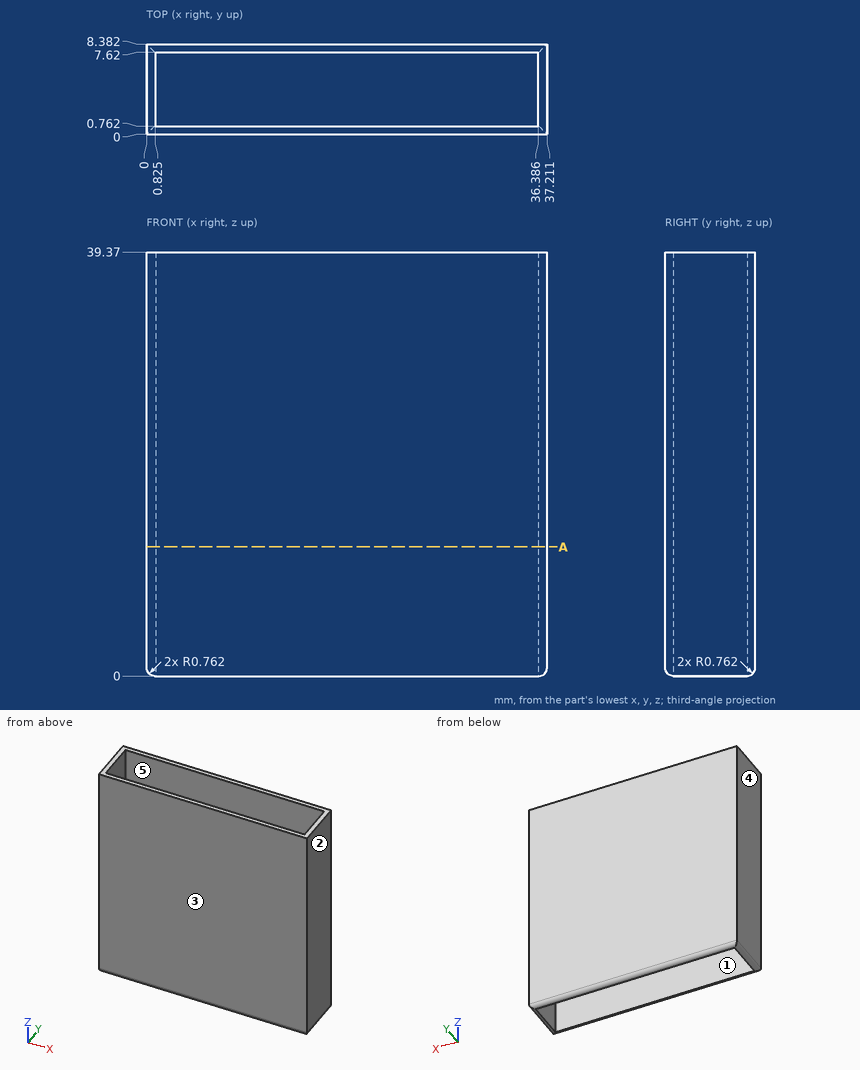
The figure shows three views and two pictorial views of one solid part (mm, origin at its lowest corner). Answer the questions. A direction names the side the tool comes from. Round coordinates to 2 decimals unless told otherwise and drop trailing zeros. Loops run counter-clockwise (first coordinate to the right, second up) from the corner with the lowest first, then second, coordinate; pieces in that order, holes last. Notation, with made-up numbers: (58, 34) - (117, 34) arc R23 cw to (117, 60) - close; hole circle Ø5 at (76.25, 48.25). An arc over 180 degrees is marked (long way). Use one line per item in the form item = value. Start each with the question number.
(1) Determine the mould class of the marked faces 1, 2 and 3 for opening direction X: +X half, -X half, draft (parallel to the pull), parting line (faces both ways), or undercut.
(2) Which of the six approach directions +Z, -Z, +X, -X, +Y, -Y give full straight-line access (tool end or side, diameter ignored) to the marked faces 4 and 5?
(3) Find section A-A on z = 12. Determine the outline of the cut face in (x, y) (1 decimal).
(4) Consider line 1 (X direction, y = 7, z = 25) (1 decimal); line 2 (Y direction, x = 12.5, z = 24.5); line 3 (Z direction, x = 22, y = 8). Determine where each line is inside the solid, lowest interval first.
(5) A flat-ended cylindrical pin translates along its axis: P1, Ø2, axis at y = 2, z = 12, coming from the -X side. Find the tip coordinate at first contact, or state that the pin passes through.
Answer list:
q1.face_1 = undercut
q1.face_2 = +X half
q1.face_3 = draft
q2.face_4 = +Z, -Z, -X, +Y, -Y
q2.face_5 = +Z, -Z
q3.outline = (0, 0) - (37.2, 0) - (37.2, 8.4) - (0, 8.4) - close; hole (0.8, 0.8) - (36.4, 0.8) - (36.4, 7.6) - (0.8, 7.6) - close
q4.line_1 = 0 to 0.8, 36.4 to 37.2
q4.line_2 = 0 to 0.76, 7.62 to 8.38
q4.line_3 = 0.1 to 39.37
q5.P1 = 0
